```python
from build123d import *

# Parameters (mm, degrees)
F1_DEPTH = 19.05
F2_DEPTH = 29.21
F3_DEPTH = 5.08
F4_W     = 10.16
F4_H     = 2.032
F5_DEPTH = 1.27
F6_SIZE  = 1.26999


# Not quite as in the source:
# - a fillet or chamfer is up to 0.001 mm smaller than in the source, because OpenCascade refuses the exact size


with BuildPart() as f1:
    # F0 (on Front) → F1 (new body)
    with BuildSketch(Plane.XZ):
        with BuildLine():
            ThreePointArc((28.575, 12.7), (26.7151280605, 17.1901280605), (22.225, 19.05))
            Line((22.225, 19.05), (-22.225, 19.05))
            ThreePointArc((-22.225, 19.05), (-26.7151280605, 17.1901280605), (-28.575, 12.7))
            Line((-28.575, 12.7), (-28.575, -12.7))
            ThreePointArc((-28.575, -12.7), (-26.7151280605, -17.1901280605), (-22.225, -19.05))
            Line((-22.225, -19.05), (22.225, -19.05))
            ThreePointArc((22.225, -19.05), (26.7151280605, -17.1901280605), (28.575, -12.7))
            Line((28.575, -12.7), (28.575, 12.7))
        make_face()
        with BuildLine():
            Line((-21.463, 17.018), (21.463, 17.018))
            ThreePointArc((21.463, 17.018), (25.0551024484, 15.5301024484), (26.543, 11.938))
            Line((26.543, 11.938), (26.543, -11.938))
            ThreePointArc((26.543, -11.938), (25.0551024484, -15.5301024484), (21.463, -17.018))
            Line((21.463, -17.018), (-21.463, -17.018))
            ThreePointArc((-21.463, -17.018), (-25.0551024484, -15.5301024484), (-26.543, -11.938))
            Line((-26.543, -11.938), (-26.543, 11.938))
            ThreePointArc((-26.543, 11.938), (-25.0551024484, 15.5301024484), (-21.463, 17.018))
        make_face(mode=Mode.SUBTRACT)
    extrude(amount=F1_DEPTH)

    # F0 (on Front) → F2 (join)
    with BuildSketch(Plane.XZ):
        with BuildLine():
            ThreePointArc((26.543, 11.938), (25.0551024484, 15.5301024484), (21.463, 17.018))
            Line((21.463, 17.018), (-21.463, 17.018))
            ThreePointArc((-21.463, 17.018), (-25.0551024484, 15.5301024484), (-26.543, 11.938))
            Line((-26.543, 11.938), (-26.543, -11.938))
            ThreePointArc((-26.543, -11.938), (-25.0551024484, -15.5301024484), (-21.463, -17.018))
            Line((-21.463, -17.018), (21.463, -17.018))
            ThreePointArc((21.463, -17.018), (25.0551024484, -15.5301024484), (26.543, -11.938))
            Line((26.543, -11.938), (26.543, 11.938))
        make_face()
        with BuildLine():
            ThreePointArc((-23.7377081066, 9.0361186621), (-22.2498105551, 12.6282211105), (-18.6577081066, 14.1161186621))
            Line((-18.6577081066, 14.1161186621), (18.6577081066, 14.1161186621))
            ThreePointArc((18.6577081066, 14.1161186621), (22.2498105551, 12.6282211105), (23.7377081066, 9.0361186621))
            Line((23.7377081066, 9.0361186621), (23.7377081066, -9.0361186621))
            ThreePointArc((23.7377081066, -9.0361186621), (22.2498105551, -12.6282211105), (18.6577081066, -14.1161186621))
            Line((18.6577081066, -14.1161186621), (-18.6577081066, -14.1161186621))
            ThreePointArc((-18.6577081066, -14.1161186621), (-22.2498105551, -12.6282211105), (-23.7377081066, -9.0361186621))
            Line((-23.7377081066, -9.0361186621), (-23.7377081066, 9.0361186621))
        make_face(mode=Mode.SUBTRACT)
    extrude(amount=F2_DEPTH)

    # F0 (on Front) → F3 (join)
    with BuildSketch(Plane.XZ):
        with BuildLine():
            Line((18.6577081066, 14.1161186621), (-18.6577081066, 14.1161186621))
            ThreePointArc((-18.6577081066, 14.1161186621), (-22.2498105551, 12.6282211105), (-23.7377081066, 9.0361186621))
            Line((-23.7377081066, 9.0361186621), (-23.7377081066, -9.0361186621))
            ThreePointArc((-23.7377081066, -9.0361186621), (-22.2498105551, -12.6282211105), (-18.6577081066, -14.1161186621))
            Line((-18.6577081066, -14.1161186621), (18.6577081066, -14.1161186621))
            ThreePointArc((18.6577081066, -14.1161186621), (22.2498105551, -12.6282211105), (23.7377081066, -9.0361186621))
            Line((23.7377081066, -9.0361186621), (23.7377081066, 9.0361186621))
            ThreePointArc((23.7377081066, 9.0361186621), (22.2498105551, 12.6282211105), (18.6577081066, 14.1161186621))
        make_face()
    extrude(amount=F3_DEPTH)

    # F4 (on face) → F5 (join)
    with BuildSketch(Plane.XY.offset(17.018)):
        with Locations((0, -24.9174)):
            Rectangle(F4_W, F4_H)
    extrude(amount=F5_DEPTH)

    # F6 (size 1.27 in the source; OpenCascade refuses exactly that, so slightly less here)
    f6_edges = [f1.edges().sort_by_distance(p)[0] for p in [
        (0, -25.9334, 18.288),
    ]]
    chamfer(f6_edges, length=F6_SIZE)


solid = f1.part
```
Work out the finished part from the listing and answer in its coordinate system (mm). A direction names the side the tool comes from. Round coordinates to 2 decimals unless told otherwise and drop trailing zeros. Order: outer loops, then holes, each group sorted by start corner. A loop starts at its lowest first (then second) coordinate and runs counter-clockwise, first axis right, second up.
Q1. A tool of negligible diameter and unlimited length cuts with its end or side. For faces 1 (the flat face through (-5.08, -24.7, 17.5)), 2 (the cylindrical face through (25.094, -24.059, 15.49)), 3 (the flat face through (0, -17, 14.116)), 4 (the flat face through (-26.543, -24, 0)), from which of +Z, -Z, +X, -X, +Y, -Y can it reach the whole face along a straight path? Write none if from no direction.
Solution:
face 1: +Z, -X, -Y
face 2: +Z, +X, -Y
face 3: -Y
face 4: +Z, -Z, -X, -Y
Q2. A cutting plane is placed at D-D, the plane y = -2.25. Determine the outline of the cut face in (x, z) (3 decimals), then the cut area to 3 significant figures.
Solution:
outline: (-28.575, -12.7) arc R6.35 ccw to (-22.225, -19.05) - (22.225, -19.05) arc R6.35 ccw to (28.575, -12.7) - (28.575, 12.7) arc R6.35 ccw to (22.225, 19.05) - (-22.225, 19.05) arc R6.35 ccw to (-28.575, 12.7) - close
area: 2,140 mm2
Q3. Find the intervals of material crossed by line 1 along X through (y, z) = (-22, 8); line 2 along Z through (x, y) = (1, -15.5), in increasing order.
Solution:
line 1: x = -26.54 to -23.74, 23.74 to 26.54
line 2: z = -19.05 to -14.12, 14.12 to 19.05
Q4. A cutting plane is placed at A-A, the plane y = -8.5. Determine the outline of the cut face in (x, z) (3 decimals), then the cut area to 3 significant figures.
Solution:
outline: (-28.575, -12.7) arc R6.35 ccw to (-22.225, -19.05) - (22.225, -19.05) arc R6.35 ccw to (28.575, -12.7) - (28.575, 12.7) arc R6.35 ccw to (22.225, 19.05) - (-22.225, 19.05) arc R6.35 ccw to (-28.575, 12.7) - close; hole (-23.738, -9.036) arc R5.08 ccw to (-18.658, -14.116) - (18.658, -14.116) arc R5.08 ccw to (23.738, -9.036) - (23.738, 9.036) arc R5.08 ccw to (18.658, 14.116) - (-18.658, 14.116) arc R5.08 ccw to (-23.738, 9.036) - close
area: 825 mm2
Q5. A cutting plane is placed at C-C, the plane x = 8. Determine the outline of the cut face in (y, z).
Solution:
outline: (-29.21, -17.02) - (-19.05, -17.02) - (-19.05, -19.05) - (0, -19.05) - (0, 19.05) - (-19.05, 19.05) - (-19.05, 17.02) - (-29.21, 17.02) - (-29.21, 14.12) - (-5.08, 14.12) - (-5.08, -14.12) - (-29.21, -14.12) - close
Q6. The mould has two halves that part along X. Classify faces 5 (the cylindrical face through (-22.21, -16.98, -12.67)), 6 (the cylindrical face through (-26.665, -9.392, 17.239)), 7 (the flat face through (5.08, -24.7, 17.5)): pulls with the +X half, pulls with the -X half, needs draft (parallel to the pull), parting line crosses it, or undercut.
Solution:
face 5: undercut
face 6: pulls with the -X half
face 7: pulls with the +X half
Q7. A cutting plane is placed at B-B, the plane z = 0. Determine the outline of the cut face in (x, y) (3 decimals), then the cut area to 3 significant figures.
Solution:
outline: (-28.575, -19.05) - (-26.543, -19.05) - (-26.543, -29.21) - (-23.738, -29.21) - (-23.738, -5.08) - (23.738, -5.08) - (23.738, -29.21) - (26.543, -29.21) - (26.543, -19.05) - (28.575, -19.05) - (28.575, 0) - (-28.575, 0) - close
area: 482 mm2
Q8. Given pin 1 Ø5 at (y, z) = (-24, 5) entering from -X; pin 2 Ø5 at (x, y) = (2, -24) entering from -Z; pin 3 Ø0.8 at (x, y) = (-1, -24.5) entering from +Z, each flat-ended and moving along its own axis, determine where each tip first touches the part or whether it passes through.
Solution:
pin 1: stops at x = -26.54
pin 2: stops at z = -17.02
pin 3: stops at z = 18.29
